from build123d import *

# Parameters (mm, degrees)
EXTRUDE_THIN1_DEPTH = 72
SKETCH2_R           = 15.24
CUT_EXTRUDE2_DEPTH  = 10
CUT_EXTRUDE3_START  = -10
SKETCH3_R           = 15.24
CUT_EXTRUDE3_DEPTH  = 10
SKETCH6_R           = 19.05
CUT_EXTRUDE4_DEPTH  = 10
FILLET2_R           = 1
FILLET3_R           = 1
FILLET4_R           = 1
FILLET5_R           = 1
FILLET6_R           = 1
FILLET7_R           = 1
FILLET8_R           = 1
FILLET9_R           = 1


with BuildPart() as part:
    # Sketch1 → Extrude-Thin1 (new body)
    with BuildSketch(Plane.XY):
        Polygon((0, 0), (60, 0), (60, -79), (0, -79), (0, -69), (50, -69), (50, -10), (0, -10), align=None)
    extrude(amount=EXTRUDE_THIN1_DEPTH)

    # Sketch2 → Cut-Extrude2 (cut)
    with BuildSketch(Plane(origin=(0, 0, 0), x_dir=(1, 0, 0), z_dir=(0, 1, 0))):
        with Locations(Location((30, -36, 0), (0, 0, 270))):
            Circle(SKETCH2_R)
    extrude(amount=-CUT_EXTRUDE2_DEPTH, mode=Mode.SUBTRACT)

    # Sketch3 → Cut-Extrude3 (cut)
    with BuildSketch(Plane.XZ.offset(79).offset(CUT_EXTRUDE3_START)):
        with Locations(Location((30, 36, 0), (0, 0, 90))):
            Circle(SKETCH3_R)
    extrude(amount=CUT_EXTRUDE3_DEPTH, mode=Mode.SUBTRACT)

    # Sketch6 → Cut-Extrude4 (cut)
    with BuildSketch(Plane.ZY.offset(-50)):
        with Locations(Location((36, -39.5, 0), (0, 0, 270))):
            Circle(SKETCH6_R)
    extrude(amount=-CUT_EXTRUDE4_DEPTH, mode=Mode.SUBTRACT)

    # Fillet2
    fillet2_edges = [part.edges().sort_by_distance(p)[0] for p in [
        (0, 0, 36),
        (30, 0, 0),
    ]]
    fillet(fillet2_edges, radius=FILLET2_R)

    # Fillet3
    fillet3_edges = [part.edges().sort_by_distance(p)[0] for p in [
        (0, -10, 36),
    ]]
    fillet(fillet3_edges, radius=FILLET3_R)

    # Fillet4
    # the kernel refuses this fillet: 1 mm, written as the material it takes off along each edge
    with BuildSketch(Plane(origin=(1, -1, 1), x_dir=(0, 0, -1), z_dir=(-1, 0, 0))) as fillet4_piece_1_section:
        Polygon((0, 0), (FILLET4_R, 0), (FILLET4_R, -FILLET4_R), (0, -FILLET4_R), align=None)
    fillet4_piece_1 = extrude(amount=FILLET4_R, mode=Mode.PRIVATE)
    fillet4_piece_1 = fillet4_piece_1 - Plane(origin=(1, -1, 1), x_dir=(0, -0.7071067811865475, 0.7071067811865475), z_dir=(-1, 0, 0)) * Sphere(FILLET4_R, mode=Mode.PRIVATE)
    add(fillet4_piece_1, mode=Mode.SUBTRACT)
    with BuildSketch(Plane(origin=(50, -10, 0), x_dir=(0, 0, 1), z_dir=(-1, 0, 0))) as fillet4_piece_2:
        with BuildLine():
            CenterArc((FILLET4_R, FILLET4_R), FILLET4_R, 180, 90)
            Line((0, FILLET4_R), (0, 0))
            Line((0, 0), (FILLET4_R, 0))
        make_face()
    extrude(amount=49, mode=Mode.SUBTRACT)
    with BuildSketch(Plane(origin=(0, -9, 0), x_dir=(0, 0, 1), z_dir=(0, 1, 0))) as fillet4_piece_3:
        with BuildLine():
            CenterArc((FILLET4_R, FILLET4_R), FILLET4_R, 180, 90)
            Line((0, FILLET4_R), (0, 0))
            Line((0, 0), (FILLET4_R, 0))
        make_face()
    extrude(amount=8, mode=Mode.SUBTRACT)
    with BuildSketch(Plane(origin=(1, -9, 0), x_dir=(-1, 0, 0), z_dir=(0, 1, 0))) as fillet4_piece_4:
        with BuildLine():
            CenterArc((1 - FILLET4_R, FILLET4_R), FILLET4_R, 270, 90)
            Line((1 - FILLET4_R, 0), (1, 0))
            Line((1, 0), (1, FILLET4_R))
        make_face()
    revolve(axis=Axis((1, -9, 0), (0, 0, 1)), revolution_arc=90, mode=Mode.SUBTRACT)

    # Fillet5
    fillet5_edges = [part.edges().sort_by_distance(p)[0] for p in [
        (30.5, 0, 72),
        (0.292893219, -0.292893219, 72),
        (25.5, -10, 72),
        (0, -5, 72),
        (0.292893219, -9.707106781, 72),
    ]]
    fillet(fillet5_edges, radius=FILLET5_R)

    # Fillet6
    fillet6_edges = [part.edges().sort_by_distance(p)[0] for p in [
        (60, -40, 0),
        (60, -0.292893219, 0.292893219),
        (60, -40, 72),
        (60, 0, 36),
        (60, -0.292893219, 71.707106781),
    ]]
    fillet(fillet6_edges, radius=FILLET6_R)

    # Fillet7
    fillet7_edges = [part.edges().sort_by_distance(p)[0] for p in [
        (0, -69, 36),
    ]]
    fillet(fillet7_edges, radius=FILLET7_R)

    # Fillet8
    fillet8_edges = [part.edges().sort_by_distance(p)[0] for p in [
        (0, -79, 36),
    ]]
    fillet(fillet8_edges, radius=FILLET8_R)

    # Fillet9
    fillet9_edges = [part.edges().sort_by_distance(p)[0] for p in [
        (0.292893219, -69.292893219, 0),
        (0.292893219, -69.292893219, 72),
        (0, -74, 0),
        (0.292893219, -78.707106781, 0),
        (0, -74, 72),
        (0.292893219, -78.707106781, 72),
        (25.5, -69, 72),
        (60, -79, 36),
        (30, -79, 0),
        (25.5, -69, 0),
        (30, -79, 72),
        (59.707106781, -79, 0.292893219),
        (59.707106781, -79, 71.707106781),
    ]]
    fillet(fillet9_edges, radius=FILLET9_R)


solid = part.part
CAD build for the part. Positions are in the model's coordinates, mm. A direction names the side the tool comes from. Round coordinates to 2 decimals unless told otherwise and drop trailing zeros. Order: outer loops, then holes, each group sorted by start corner. A loop starts at its lowest first (then second) coordinate and runs counter-clockwise, first axis right, second up. Notation, with made-up numbers: (-2.5, -23.75) - (37.5, -23.75) arc R13 ccw to (37.5, -6.75) - close; hole circle Ø1 at (-40, 8). An arc over 180 degrees is marked (long way). Return JSON: item names as keys, results as strings.
(1) Cut at D-D (y = -5). Give the cut face in (x, z).
Answer key:
{"outline": "(0, 1) arc R1 ccw to (1, 0) - (59, 0) arc R1 ccw to (60, 1) - (60, 71) arc R1 ccw to (59, 72) - (1, 72) arc R1 ccw to (0, 71) - close; hole circle Ø30.48 at (30, 36)"}
(2) Pull direction Z, two halves, no side cores. Call faces 1 (the face through (60, -22, 28)), 2 (the face through (54.93, -57.67, 41.72)), 3 (the face through (52, -42, 72)): +Z half, -Z half, draft (parallel to the pull), parting line (faces both ways), or undercut.
Answer key:
{"face 1": "draft", "face 2": "undercut", "face 3": "+Z half"}
(3) Tool access for faces 4 (the face through (15, -10, 28)), 5 (the face through (0, -5, 36)): list every direction of +Z, -Z, +X, -X, +Y, -Y with a clear straight run to the whole face (end or side of a thin tool).
Answer key:
{"face 4": "+Z, -Z, -X", "face 5": "+Z, -Z, -X, +Y, -Y"}
(4) Cut at C-C (z = 36). Give the cut face in (x, y), then the cut area to 3 significant figures.
Answer key:
{"outline": "(0, -78) arc R1 ccw to (1, -79) - (14.76, -79) - (14.76, -69) - (1, -69) arc R1 ccw to (0, -70) - close; (0, -9) arc R1 ccw to (1, -10) - (14.76, -10) - (14.76, 0) - (1, 0) arc R1 ccw to (0, -1) - close; (45.24, -79) - (59, -79) arc R1 ccw to (60, -78) - (60, -58.55) - (50, -58.55) - (50, -69) - (45.24, -69) - close; (45.24, -10) - (50, -10) - (50, -20.45) - (60, -20.45) - (60, -1) arc R1 ccw to (59, 0) - (45.24, 0) - close", "area": "798 mm^2"}
(5) Wall check: probe 1 along X at (y, z) = (-3.25, 36); probe 2 along Y at (x, z) = (45, 6); probe 3 along Z at (x, y) = (57, -39). Give the ranges that are in metal, low to high. Write a range as from..to.
Answer key:
{"probe 1": "x = 0..14.76, 45.24..60", "probe 2": "y = -79..-69, -10..0", "probe 3": "z = 0..16.96, 55.04..72"}
(6) Pin check, flat tip, straight feed: pin 1 Ø6 at (x, y) = (40, -10.5) entering from -Z. Stop position of the tip, or through.
Answer key:
{"pin 1": "stops at z = 0"}
(7) Cut at B-B (y = -39.5). Give the cut face in (x, z), then the cut area to 3 significant figures.
Answer key:
{"outline": "(50, 0) - (59, 0) arc R1 ccw to (60, 1) - (60, 16.95) - (50, 16.95) - close; (50, 55.05) - (60, 55.05) - (60, 71) arc R1 ccw to (59, 72) - (50, 72) - close", "area": "339 mm^2"}
(8) Cut at A-A (x = 30). Give the cut face in (y, z), then the cut area to 3 significant figures.
Answer key:
{"outline": "(-79, 1) arc R1 ccw to (-78, 0) - (-70, 0) arc R1 ccw to (-69, 1) - (-69, 20.76) - (-79, 20.76) - close; (-79, 51.24) - (-69, 51.24) - (-69, 71) arc R1 ccw to (-70, 72) - (-78, 72) arc R1 ccw to (-79, 71) - close; (-10, 1) arc R1 ccw to (-9, 0) - (-1, 0) arc R1 ccw to (0, 1) - (0, 20.76) - (-10, 20.76) - close; (-10, 51.24) - (0, 51.24) - (0, 71) arc R1 ccw to (-1, 72) - (-9, 72) arc R1 ccw to (-10, 71) - close", "area": "829 mm^2"}
